Part model, mm, in its own coordinate system. A direction names the side the tool comes from. Coordinates: 2 decimals unless noted, no trailing zeros. Order: outer loops, then holes, each group sorted by start corner. A loop starts at its lowest first (then second) coordinate and runs counter-clockwise, first axis right, second up.
1) Cut at A-A (z = 15.5). List the corners of the cut face in (x, y), and give its area (3 significant figures).
2) Pin check, flat tips, straight feed: pin 1 Ø3 at (x, z) = (77, 0.5) entering from +Y; pin 2 Ø1 at (x, y) = (-14, 1) entering from +Z. Stop position of each tip, or through.
3) Cut at B-B (y = 1.55). Give the number of separate pieces and of enclosed holes in the cut face, and give its area (3 significant figures).
4) Cut at C-C (x = 44.5). List the corners of the cut face in (y, z).
5) Wall check: L1, parallel to Z at x = 81, y = 0.1; L2, parallel to Z at x = 95, y = 0.8; L3, parallel to Z at x = 81.25, y = 0.5. Give the ranges that are in metal, low to high.
6) Mould opens along X. For faces 1 (the flat face through (97.63, 0.99, 27.46)), 2 (the flat face through (45.712, 0.986, 4.437)), 3 (the flat face through (-19.97, 0.99, 37.79)) say: +X half, -X half, draft (parallel to the pull), parting line (faces both ways), or undercut.
7) Tool access for faces 4 (the flat face through (53.92, 0.99, 10.48)), 5 (the flat face through (47.58, 0.99, 39.48)), 6 (the cylindrical face through (15, 1, 12.9)): list every direction of +Z, -Z, +X, -X, +Y, -Y with a clear straight run to the whole face (end or side of a thin tool).
```python
from build123d import *

# Parameters (mm, degrees)
SKETCH1_R           = 1.75
SKETCH1_R_2         = 1.5
SKETCH1_R_3         = 5
BOSS_EXTRUDE1_DEPTH = 2


with BuildPart() as part:
    # Sketch1 → Boss-Extrude1 (new body)
    with BuildSketch(Plane(origin=(0, 0, 0), x_dir=(1, 0, 0), z_dir=(0, 1, 0))):
        with BuildLine():
            Line((0, 0), (43, 0))
            Line((43, 0), (48.5, -9))
            Line((48.5, -9), (59.5, -12))
            Line((59.5, -12), (69.5, -12))
            Line((69.5, -12), (74.5, 2.5))
            Line((74.5, 2.5), (101.5, -0.5))
            Line((101.5, -0.5), (107, -9.5))
            Line((107, -9.5), (107, -24.5))
            Line((107, -24.5), (88, -30.5))
            Line((88, -30.5), (85.5, -34.5))
            ThreePointArc((85.5, -34.5), (82.533474843, -40.320323174), (76.870377201, -37.063674828))
            Line((76.870377201, -37.063674828), (74, -35))
            Line((74, -35), (63, -38))
            Line((63, -38), (53, -38))
            Line((53, -38), (42, -41))
            Line((42, -41), (34, -41))
            Line((34, -41), (23, -31.5))
            Line((23, -31.5), (-5, -31.5))
            Line((-5, -31.5), (-7, -40.5))
            Line((-7, -40.5), (-18, -40.5))
            Line((-18, -40.5), (-22, -35))
            Line((-22, -35), (-22, -24))
            Line((-22, -24), (-16, -10))
            Line((-16, -10), (-6, -8))
            Line((-6, -8), (0, 0))
        make_face()
        with Locations(Location((40.25, -36, 0), (0, 0, 270))):
            Circle(SKETCH1_R, mode=Mode.SUBTRACT)
        with Locations(Location((81.25, -36, 0), (0, 0, 270))):
            Circle(SKETCH1_R_2, mode=Mode.SUBTRACT)
        with Locations(Location((91, -16.5, 0), (0, 0, 270))):
            Circle(SKETCH1_R_3, mode=Mode.SUBTRACT)
        with Locations(Location((77, -0.5, 0), (0, 0, 270))):
            Circle(SKETCH1_R, mode=Mode.SUBTRACT)
        with Locations(Location((81, -9.5, 0), (0, 0, 270))):
            Circle(SKETCH1_R_2, mode=Mode.SUBTRACT)
        with Locations(Location((100, -2.5, 0), (0, 0, 270))):
            Circle(SKETCH1_R_2, mode=Mode.SUBTRACT)
        with Locations(Location((102, -19.75, 0), (0, 0, 270))):
            Circle(SKETCH1_R_2, mode=Mode.SUBTRACT)
        with Locations(Location((53, -19, 0), (0, 0, 270))):
            Circle(SKETCH1_R_2, mode=Mode.SUBTRACT)
        with Locations(Location((34.25, -19, 0), (0, 0, 270))):
            Circle(SKETCH1_R_2, mode=Mode.SUBTRACT)
        with Locations(Location((13.5, -12, 0), (0, 0, 270))):
            Circle(SKETCH1_R, mode=Mode.SUBTRACT)
        with BuildLine():
            Line((-16, -34.5), (-11.5, -34.5))
            ThreePointArc((-11.5, -34.5), (-10, -36), (-11.5, -37.5))
            Line((-11.5, -37.5), (-16, -37.5))
            ThreePointArc((-16, -37.5), (-17.5, -36), (-16, -34.5))
        make_face(mode=Mode.SUBTRACT)
    extrude(amount=BOSS_EXTRUDE1_DEPTH)


solid = part.part
```
Geometry check:
1. outline: (-18.36, 0) - (86.1, 0) - (86.1, 2) - (-18.36, 2) - close; (95.9, 0) - (107, 0) - (107, 2) - (95.9, 2) - close
1. area: 231 mm2
2. pin 1: passes through
2. pin 2: stops at z = 40.5
3. separate pieces: 1
3. enclosed holes: 11
3. area: 3,870 mm2
4. outline: (0, 2.45) - (2, 2.45) - (2, 40.32) - (0, 40.32) - close
5. L1: z = -1.78 to 8, 11 to 34.52, 37.48 to 40.5
5. L2: z = -0.22 to 13.5, 19.5 to 28.29
5. L3: z = -1.75 to 8.02, 10.98 to 34.5, 37.5 to 40.51
6. face 1: +X half
6. face 2: undercut
6. face 3: -X half
7. face 4: -Z, +Y, -Y
7. face 5: +Z, +Y, -Y
7. face 6: +Y, -Y
